Here's the drawing with two shaded views (mm, measured from the low corner). I have some questions. Round coordinates to 2 decimals unless told otherwise and drop trailing zeros. Write each loop counter-clockwise with the first axis right and the second up, starting at its lowest first coordinate (ties: lowest second). Pieces come first, ordered by that corner, then holes. Notation, with made-up numbers: M 14,-24.75 L 41,-24.75 A12 ccw 41,-8.75 Z; hole C 7.5,78 d3. An arc over 180 degrees is marked long. Use one line per item in the form item = value. Start each with the question number.
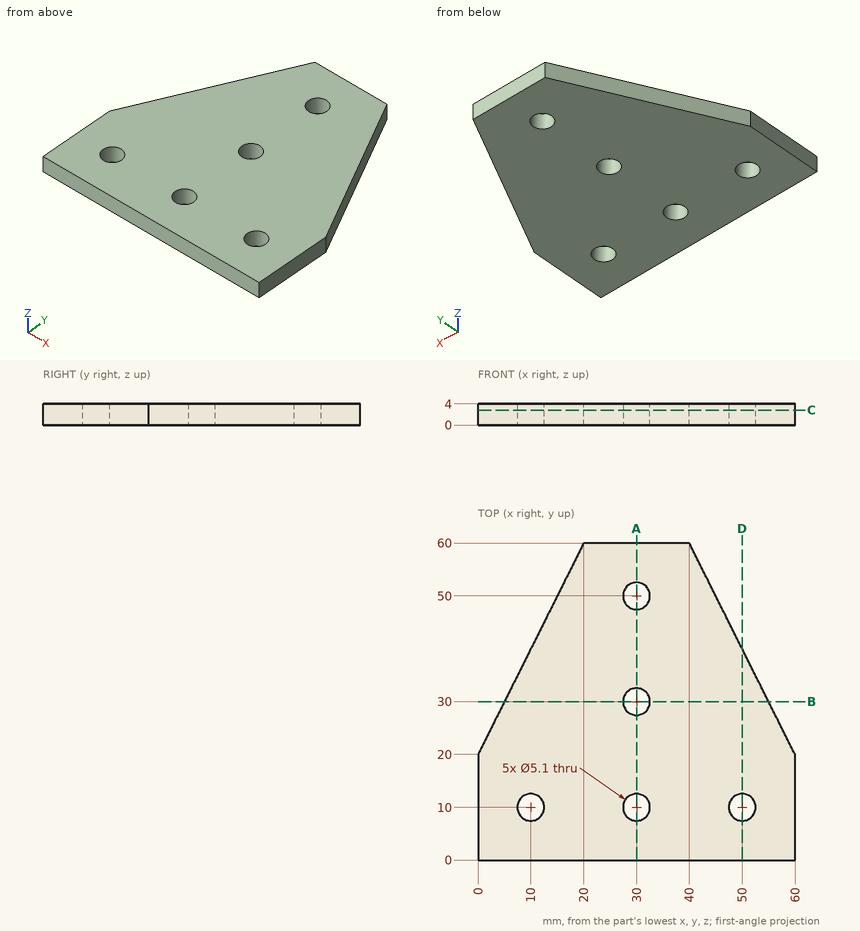
1. Please list where these lines run through material, in increasing order: line 1 along Y through (x, z) = (30, 2.9); line 2 along Y through (x, z) = (28.5, 3.7); line 3 along Y through (x, z) = (50, 1.35).
2. If we section it at D-D (x = 50): List the corners of the cut face in (y, z) for me.
3. If we section it at A-A (x = 30): List the corners of the cut face in (y, z) for me.
4. If we section it at B-B (y = 30): List the corners of the cut face in (x, z) for me.
5. If we section it at C-C (z = 2.85): List the corners of the cut face in (x, y) for me.
6. Will these pins go through, and if not, where does the flat tip stop? pin 1 (8 mm diameter, centred on x = 50, y = 10, fed in from +Z); pin 2 (3 mm diameter, centred on x = 30, y = 10, fed in from -Z); pin 3 (1 mm diameter, centred on y = 47.5, z = 1, fed in from +X); pin 4 (2 mm diameter, centred on y = 41.5, z = 1, fed in from -X).
Model answer:
q1.line_1 = 0 to 7.45, 12.55 to 27.45, 32.55 to 47.45, 52.55 to 60
q1.line_2 = 0 to 7.94, 12.06 to 27.94, 32.06 to 47.94, 52.06 to 60
q1.line_3 = 0 to 7.45, 12.55 to 40
q2.outline = M 0,0 L 7.45,0 L 7.45,4 L 0,4 Z; M 12.55,0 L 40,0 L 40,4 L 12.55,4 Z
q3.outline = M 0,0 L 7.45,0 L 7.45,4 L 0,4 Z; M 12.55,0 L 27.45,0 L 27.45,4 L 12.55,4 Z; M 32.55,0 L 47.45,0 L 47.45,4 L 32.55,4 Z; M 52.55,0 L 60,0 L 60,4 L 52.55,4 Z
q4.outline = M 5,0 L 27.45,0 L 27.45,4 L 5,4 Z; M 32.55,0 L 55,0 L 55,4 L 32.55,4 Z
q5.outline = M 0,0 L 60,0 L 60,20 L 40,60 L 20,60 L 0,20 Z; hole C 10,10 d5.1; hole C 30,10 d5.1; hole C 30,30 d5.1; hole C 30,50 d5.1; hole C 50,10 d5.1
q6.pin_1 = 4
q6.pin_2 = through
q6.pin_3 = 46.5
q6.pin_4 = 10.25
